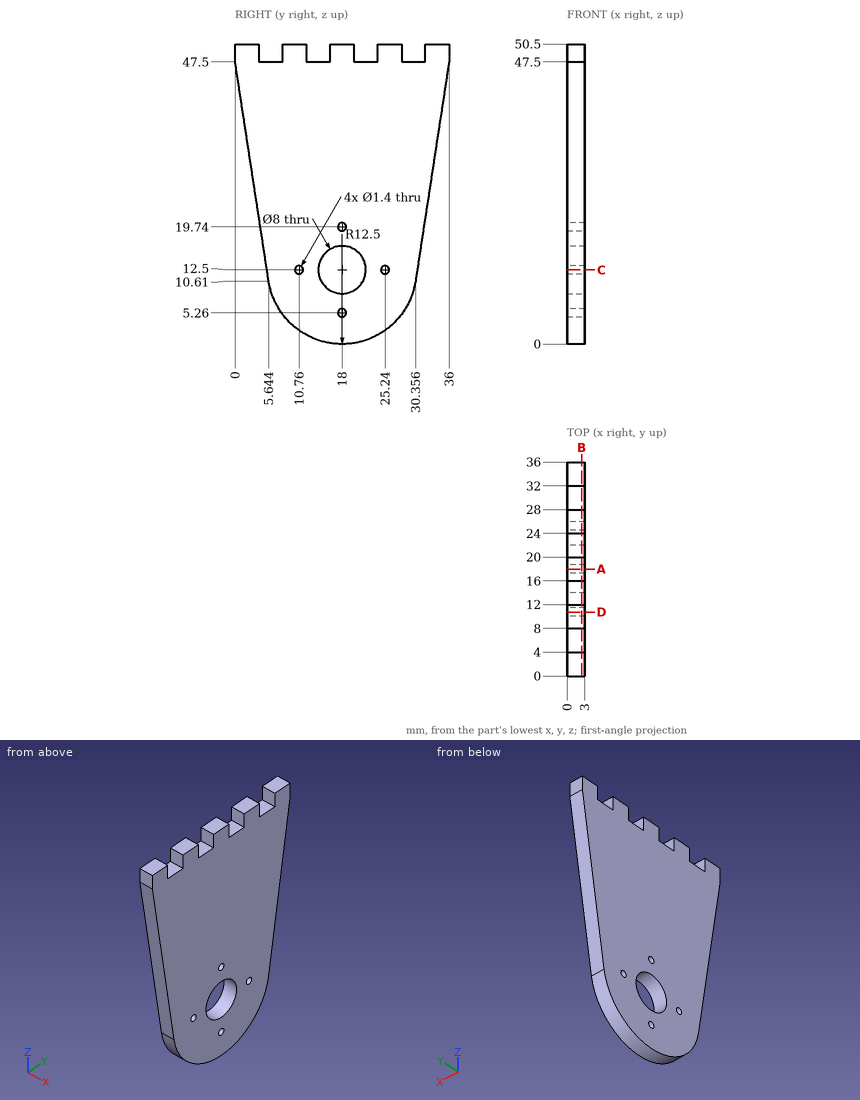
For this review, use the dimensioned drawing (mm, ordinates from the lowest corner) and the shaded views. Coordinates: 2 decimals unless noted, no trailing zeros. Write each loop counter-clockwise with the first axis right and the second up, starting at its lowest first coordinate (ties: lowest second). Pieces come first, ordered by that corner, then holes. Notation, with made-up numbers: (72.25, -1.5) -> (96.25, -1.5) arc R22 ccw to (96.25, 27.5) -> close; hole circle Ø5 at (57.25, 89). An arc over 180 degrees is marked (long way). Write each question's results on one line, items separated by ' | '. Start each with the question number.
(1) Take a section at B-B on x = 2.45. Write out the cut boundary in (y, z), and give its area (3 significant figures).
(2) Take a section at A-A on y = 18. Write out the cut boundary in (x, z), and give its area (3 significant figures).
(3) Take a section at C-C on z = 12.5. Write out the cut boundary in (x, y) (1 decimal).
(4) For line 1 along Z through (x, y) = (0.25, 17); line 2 along Z through (x, y) = (2.7, 19.5); line 3 along Y through (x, z) = (1.65, 12.5) (1 decimal), list the stretches that pass through material, from the lowest coordinate up. Write a range as from..to.
(5) Take a section at D-D on y = 10.76. Write out the cut boundary in (x, z), and give its area (3 significant figures).
(6) Clearance check with flat-ended pins moving along their axes: P1, Ø1.3, axis at y = 18, z = 19.74, coming from the +X side; P2, Ø1.5, axis at x = 1, y = 21, coming from the +Z side. State where each tip first meets the part, or that it passes through.
Results found:
1) outline: (0, 47.5) -> (5.64, 10.61) arc R12.5 ccw to (30.36, 10.61) -> (36, 47.5) -> (36, 50.5) -> (32, 50.5) -> (32, 47.5) -> (28, 47.5) -> (28, 50.5) -> (24, 50.5) -> (24, 47.5) -> (20, 47.5) -> (20, 50.5) -> (16, 50.5) -> (16, 47.5) -> (12, 47.5) -> (12, 50.5) -> (8, 50.5) -> (8, 47.5) -> (4, 47.5) -> (4, 50.5) -> (0, 50.5) -> close; hole circle Ø1.4 at (10.76, 12.5); hole circle Ø8 at (18, 12.5); hole circle Ø1.4 at (18, 5.26); hole circle Ø1.4 at (18, 19.74); hole circle Ø1.4 at (25.24, 12.5) | area: 1,320 mm2
2) outline: (0, 0) -> (3, 0) -> (3, 4.56) -> (0, 4.56) -> close; (0, 5.96) -> (3, 5.96) -> (3, 8.5) -> (0, 8.5) -> close; (0, 16.5) -> (3, 16.5) -> (3, 19.04) -> (0, 19.04) -> close; (0, 20.44) -> (3, 20.44) -> (3, 50.5) -> (0, 50.5) -> close | area: 119 mm2
3) outline: (0, 5.4) -> (3, 5.4) -> (3, 10.1) -> (0, 10.1) -> close; (0, 11.5) -> (3, 11.5) -> (3, 14) -> (0, 14) -> close; (0, 22) -> (3, 22) -> (3, 24.5) -> (0, 24.5) -> close; (0, 25.9) -> (3, 25.9) -> (3, 30.6) -> (0, 30.6) -> close
4) line 1: z = 0.04..8.63, 16.37..50.5 | line 2: z = 0.09..8.79, 16.21..50.5 | line 3: y = 5.4..10.1, 11.5..14, 22..24.5, 25.9..30.6
5) outline: (0, 2.31) -> (3, 2.31) -> (3, 11.8) -> (0, 11.8) -> close; (0, 13.2) -> (3, 13.2) -> (3, 50.5) -> (0, 50.5) -> close | area: 140 mm2
6) P1: passes through | P2: stops at z = 47.5
